from build123d import *

# Parameters (mm, degrees)
SKETCH1_W           = 50
SKETCH1_H           = 50
BOSS_EXTRUDE1_DEPTH = 25
SKETCH2_R           = 3
SKETCH2_W           = 34
SKETCH2_H           = 34
CUT_EXTRUDE1_DEPTH  = 18
CHAMFER1_SIZE       = 2
CHAMFER2_SIZE       = 1
FILLET1_R           = 2
CHAMFER3_SIZE       = 0.5


with BuildPart() as part:
    # Sketch1 → Boss-Extrude1 (new body)
    with BuildSketch(Plane(origin=(0, 0, 0), x_dir=(1, 0, 0), z_dir=(0, 1, 0))):
        Rectangle(SKETCH1_W, SKETCH1_H)
    extrude(amount=BOSS_EXTRUDE1_DEPTH)

    # Sketch2 → Cut-Extrude1 (cut)
    with BuildSketch(Plane(origin=(0, 25, 0), x_dir=(1, 0, 0), z_dir=(0, 1, 0))):
        with Locations(Location((-19.568429399, -20.066458938, 0), (0, 0, 270))):
            Circle(SKETCH2_R)
        with Locations(Location((-19.410173636, 20.192344443, 0), (0, 0, 270))):
            Circle(SKETCH2_R)
        with Locations(Location((19.591857754, -20.046682357, 0), (0, 0, 270))):
            Circle(SKETCH2_R)
        with Locations(Location((19.434027978, 20.17419404, 0), (0, 0, 270))):
            Circle(SKETCH2_R)
        Rectangle(SKETCH2_W, SKETCH2_H)
    extrude(amount=-CUT_EXTRUDE1_DEPTH, mode=Mode.SUBTRACT)

    # Chamfer1
    chamfer1_edges = [part.edges().sort_by_distance(p)[0] for p in [
        (0, 0, 25),
        (-25, 0, 0),
        (0, 0, -25),
        (25, 0, 0),
        (25, 12.5, 25),
        (-25, 12.5, 25),
        (-25, 12.5, -25),
        (25, 12.5, -25),
    ]]
    chamfer(chamfer1_edges, length=CHAMFER1_SIZE)

    # Chamfer2
    chamfer2_edges = [part.edges().sort_by_distance(p)[0] for p in [
        (-25, 25, 0),
        (0, 25, -25),
        (0, 25, 25),
        (25, 25, 0),
    ]]
    chamfer(chamfer2_edges, length=CHAMFER2_SIZE - 0.0001)  # a hair under: the kernel refuses the full size

    # Fillet1
    fillet1_edges = [part.edges().sort_by_distance(p)[0] for p in [
        (17, 16, 17),
        (-17, 16, 17),
        (-17, 16, -17),
        (17, 16, -17),
    ]]
    fillet(fillet1_edges, radius=FILLET1_R)

    # Chamfer3
    chamfer3_edges = [part.edges().sort_by_distance(p)[0] for p in [
        (19.591857754, 25, 17.046682357),
        (19.434027978, 25, -23.17419404),
        (-19.410173636, 25, -23.192344443),
        (-19.568429399, 25, 17.066458938),
    ]]
    chamfer(chamfer3_edges, length=CHAMFER3_SIZE)


solid = part.part
Model file for the job. Use its own axes, mm. A direction names the side the tool comes from. Give positions to 0.01 mm unless a question says otherwise; leave off trailing zeros. Order: outer loops, then holes, each group sorted by start corner. A loop starts at its lowest first (then second) coordinate and runs counter-clockwise, first axis right, second up. Notation, with made-up numbers: (-20, -29) - (0, -29) arc R12 ccw to (0, -8) - close; hole circle Ø11 at (-31.75, 79). An arc over 180 degrees is marked (long way). Write item = value, one per line. Start each with the question number.
1. Which spindle directions (+Z, -Z, +X, -X, +Y, -Y) get a long thin tool onto all of the face, cutting with end or side? Do faces 1 (the flat face through (23.8, 1.4, 23.6)), 2 (the flat face through (-19, 7, -20)). Say none if no direction does.
2. Drop a flat-ended pin along its axis: P1, Ø5, axis at x = 19.43, z = -20.17, coming from the +Y side. Give the stop position or say it passes through.
3. Cut at B-B, the plane z = -8.5. List the corners of the cut face in (x, y), and give its area (3 significant figures).
4. Cut at A-A, the plane x = -4.5. List the corners of the cut face in (y, z), and give its area (3 significant figures).
5. Cut at C-C, the plane y = 18. List the corners of the cut face in (x, z).
6. Probe line 1 along Z through (x, y) = (-19.5, 20); line 2 along Z through (x, y) = (-8, 13.5). List the from-to ranges inside material, lowest first.
7. Two-plate mould, pull along Z, no slides. Class faces 3 (the flat face through (-24, 1, 0)), 4 (the flat face through (0, 16, 17)), 5 (the flat face through (0, 1, 24)): pulls with the +Z half, pulls with the -Z half, needs draft (parallel to the pull), parting line crosses it, or undercut.
Taken from the geometry:
q1.face_1 = +Z, +X, -Y
q1.face_2 = +Y
q2.P1 = 7
q3.outline = (-25, 2) - (-23, 0) - (23, 0) - (25, 2) - (25, 24) - (24, 25) - (17, 25) - (17, 7) - (-17, 7) - (-17, 25) - (-24, 25) - (-25, 24) - close
q3.area = 633 mm²
q4.outline = (0, -23) - (2, -25) - (24, -25) - (25, -24) - (25, -17) - (7, -17) - (7, 17) - (25, 17) - (25, 24) - (24, 25) - (2, 25) - (0, 23) - close
q4.area = 633 mm²
q5.outline = (-25, -23) - (-23, -25) - (23, -25) - (25, -23) - (25, 23) - (23, 25) - (-23, 25) - (-25, 23) - close; hole circle Ø6 at (-19.57, 20.07); hole circle Ø6 at (-19.41, -20.19); hole (-17, -15) arc R2 ccw to (-15, -17) - (15, -17) arc R2 ccw to (17, -15) - (17, 15) arc R2 ccw to (15, 17) - (-15, 17) arc R2 ccw to (-17, 15) - close; hole circle Ø6 at (19.43, -20.17); hole circle Ø6 at (19.59, 20.05)
q6.line_1 = -25 to -23.19, -17.19 to 17.07, 23.07 to 25
q6.line_2 = -25 to -17, 17 to 25
q7.face_3 = needs draft
q7.face_4 = undercut
q7.face_5 = pulls with the +Z half
